from build123d import *

# Parameters (mm, degrees)
ESQUISSE1_W                  = 300
ESQUISSE1_H                  = 100
BOSS_EXTRU_1_DEPTH           = 1.5875
ESQUISSE2_W                  = 19.05
ESQUISSE2_H                  = 61.9
BOSS_EXTRU_2_DEPTH           = 1.5875
ESQUISSE3_W                  = 1.5875
ESQUISSE3_H                  = 61.9
BOSS_EXTRU_3_DEPTH           = 17.4625
ENL_V_MAT_EXTRU_1_REACH      = 5.175
ESQUISSE4_R                  = 1.5875
ENL_V_MAT_EXTRU_2_REACH      = 22.637
ESQUISSE5_R                  = 1.5875
ESQUISSE7_R                  = 1.5875
ENL_V_MAT_EXTRU_4_DEPTH      = 297.825
ENL_V_MAT_EXTRU_4_DEPTH_BACK = 4.175
ESQUISSE8_R                  = 1.5875
ENL_V_MAT_EXTRU_5_DEPTH      = 1.5875


with BuildPart() as part:
    # Esquisse1 → Boss.-Extru.1 (new body)
    with BuildSketch(Plane.XY):
        with Locations((29.89832913, 31.147540984)):
            Rectangle(ESQUISSE1_W, ESQUISSE1_H)
    extrude(amount=BOSS_EXTRU_1_DEPTH)

    # Esquisse2 → Boss.-Extru.2 (add)
    with BuildSketch(Plane(origin=(0, 0, 0), x_dir=(-1, 0, 0), z_dir=(0, 0, -1))):
        with Locations((108.98917087, 31.147540984)):
            Rectangle(ESQUISSE2_W, ESQUISSE2_H)
        with Locations((-168.78582913, 31.147540984)):
            Rectangle(ESQUISSE2_W, ESQUISSE2_H)
    extrude(amount=BOSS_EXTRU_2_DEPTH)

    # Esquisse3 → Boss.-Extru.3 (add)
    with BuildSketch(Plane(origin=(0, 0, -1.5875), x_dir=(-1, 0, 0), z_dir=(0, 0, -1))):
        with Locations((-177.51707913, 31.147540984)):
            Rectangle(ESQUISSE3_W, ESQUISSE3_H)
        with Locations((117.72042087, 31.147540984)):
            Rectangle(ESQUISSE3_W, ESQUISSE3_H)
    extrude(amount=BOSS_EXTRU_3_DEPTH)

    # Esquisse4 → Enlèv. mat.-Extru.1 (cut, up to next)
    with BuildSketch(Plane(origin=(0, 0, -1.5875), x_dir=(-1, 0, 0), z_dir=(0, 0, -1)), mode=Mode.PRIVATE) as enl_v_mat_extru_1_sk1:
        with Locations((-167.99207913, 52.572540984)):
            Circle(ESQUISSE4_R)
    enl_v_mat_extru_1_tool1 = extrude(enl_v_mat_extru_1_sk1.sketch, amount=-ENL_V_MAT_EXTRU_1_REACH, mode=Mode.PRIVATE) & part.part
    add(enl_v_mat_extru_1_tool1.solids().sort_by_distance((167.992079, 52.572541, -1.5875))[0], mode=Mode.SUBTRACT)
    # Esquisse4 → Enlèv. mat.-Extru.1 (cut, up to next)
    with BuildSketch(Plane(origin=(0, 0, -1.5875), x_dir=(-1, 0, 0), z_dir=(0, 0, -1)), mode=Mode.PRIVATE) as enl_v_mat_extru_1_sk2:
        with Locations((-167.99207913, 9.722540984)):
            Circle(ESQUISSE4_R)
    enl_v_mat_extru_1_tool2 = extrude(enl_v_mat_extru_1_sk2.sketch, amount=-ENL_V_MAT_EXTRU_1_REACH, mode=Mode.PRIVATE) & part.part
    add(enl_v_mat_extru_1_tool2.solids().sort_by_distance((167.992079, 9.722541, -1.5875))[0], mode=Mode.SUBTRACT)
    # Esquisse4 → Enlèv. mat.-Extru.1 (cut, up to next)
    with BuildSketch(Plane(origin=(0, 0, -1.5875), x_dir=(-1, 0, 0), z_dir=(0, 0, -1)), mode=Mode.PRIVATE) as enl_v_mat_extru_1_sk3:
        with Locations((108.19542087, 52.572540984)):
            Circle(ESQUISSE4_R)
    enl_v_mat_extru_1_tool3 = extrude(enl_v_mat_extru_1_sk3.sketch, amount=-ENL_V_MAT_EXTRU_1_REACH, mode=Mode.PRIVATE) & part.part
    add(enl_v_mat_extru_1_tool3.solids().sort_by_distance((-108.195421, 52.572541, -1.5875))[0], mode=Mode.SUBTRACT)
    # Esquisse4 → Enlèv. mat.-Extru.1 (cut, up to next)
    with BuildSketch(Plane(origin=(0, 0, -1.5875), x_dir=(-1, 0, 0), z_dir=(0, 0, -1)), mode=Mode.PRIVATE) as enl_v_mat_extru_1_sk4:
        with Locations((108.19542087, 9.722540984)):
            Circle(ESQUISSE4_R)
    enl_v_mat_extru_1_tool4 = extrude(enl_v_mat_extru_1_sk4.sketch, amount=-ENL_V_MAT_EXTRU_1_REACH, mode=Mode.PRIVATE) & part.part
    add(enl_v_mat_extru_1_tool4.solids().sort_by_distance((-108.195421, 9.722541, -1.5875))[0], mode=Mode.SUBTRACT)

    # Esquisse5 → Enlèv. mat.-Extru.2 (cut, up to next)
    with BuildSketch(Plane.XY.offset(1.5875), mode=Mode.PRIVATE) as enl_v_mat_extru_2_sk1:
        with Locations((-108.19542087, -8.533709016)):
            Circle(ESQUISSE5_R)
    enl_v_mat_extru_2_tool1 = extrude(enl_v_mat_extru_2_sk1.sketch, amount=-ENL_V_MAT_EXTRU_2_REACH, mode=Mode.PRIVATE) & part.part
    add(enl_v_mat_extru_2_tool1.solids().sort_by_distance((-108.195421, -8.533709, 1.5875))[0], mode=Mode.SUBTRACT)
    # Esquisse5 → Enlèv. mat.-Extru.2 (cut, up to next)
    with BuildSketch(Plane.XY.offset(1.5875), mode=Mode.PRIVATE) as enl_v_mat_extru_2_sk2:
        with Locations((-89.93917087, -8.533709016)):
            Circle(ESQUISSE5_R)
    enl_v_mat_extru_2_tool2 = extrude(enl_v_mat_extru_2_sk2.sketch, amount=-ENL_V_MAT_EXTRU_2_REACH, mode=Mode.PRIVATE) & part.part
    add(enl_v_mat_extru_2_tool2.solids().sort_by_distance((-89.939171, -8.533709, 1.5875))[0], mode=Mode.SUBTRACT)
    # Esquisse5 → Enlèv. mat.-Extru.2 (cut, up to next)
    with BuildSketch(Plane.XY.offset(1.5875), mode=Mode.PRIVATE) as enl_v_mat_extru_2_sk3:
        with Locations((-30.02042087, -8.533709016)):
            Circle(ESQUISSE5_R)
    enl_v_mat_extru_2_tool3 = extrude(enl_v_mat_extru_2_sk3.sketch, amount=-ENL_V_MAT_EXTRU_2_REACH, mode=Mode.PRIVATE) & part.part
    add(enl_v_mat_extru_2_tool3.solids().sort_by_distance((-30.020421, -8.533709, 1.5875))[0], mode=Mode.SUBTRACT)
    # Esquisse5 → Enlèv. mat.-Extru.2 (cut, up to next)
    with BuildSketch(Plane.XY.offset(1.5875), mode=Mode.PRIVATE) as enl_v_mat_extru_2_sk4:
        with Locations((29.89832913, -8.533709016)):
            Circle(ESQUISSE5_R)
    enl_v_mat_extru_2_tool4 = extrude(enl_v_mat_extru_2_sk4.sketch, amount=-ENL_V_MAT_EXTRU_2_REACH, mode=Mode.PRIVATE) & part.part
    add(enl_v_mat_extru_2_tool4.solids().sort_by_distance((29.898329, -8.533709, 1.5875))[0], mode=Mode.SUBTRACT)
    # Esquisse5 → Enlèv. mat.-Extru.2 (cut, up to next)
    with BuildSketch(Plane.XY.offset(1.5875), mode=Mode.PRIVATE) as enl_v_mat_extru_2_sk5:
        with Locations((89.81707913, -8.533709016)):
            Circle(ESQUISSE5_R)
    enl_v_mat_extru_2_tool5 = extrude(enl_v_mat_extru_2_sk5.sketch, amount=-ENL_V_MAT_EXTRU_2_REACH, mode=Mode.PRIVATE) & part.part
    add(enl_v_mat_extru_2_tool5.solids().sort_by_distance((89.817079, -8.533709, 1.5875))[0], mode=Mode.SUBTRACT)
    # Esquisse5 → Enlèv. mat.-Extru.2 (cut, up to next)
    with BuildSketch(Plane.XY.offset(1.5875), mode=Mode.PRIVATE) as enl_v_mat_extru_2_sk6:
        with Locations((149.73582913, -8.533709016)):
            Circle(ESQUISSE5_R)
    enl_v_mat_extru_2_tool6 = extrude(enl_v_mat_extru_2_sk6.sketch, amount=-ENL_V_MAT_EXTRU_2_REACH, mode=Mode.PRIVATE) & part.part
    add(enl_v_mat_extru_2_tool6.solids().sort_by_distance((149.735829, -8.533709, 1.5875))[0], mode=Mode.SUBTRACT)
    # Esquisse5 → Enlèv. mat.-Extru.2 (cut, up to next)
    with BuildSketch(Plane.XY.offset(1.5875), mode=Mode.PRIVATE) as enl_v_mat_extru_2_sk7:
        with Locations((167.99207913, -8.533709016)):
            Circle(ESQUISSE5_R)
    enl_v_mat_extru_2_tool7 = extrude(enl_v_mat_extru_2_sk7.sketch, amount=-ENL_V_MAT_EXTRU_2_REACH, mode=Mode.PRIVATE) & part.part
    add(enl_v_mat_extru_2_tool7.solids().sort_by_distance((167.992079, -8.533709, 1.5875))[0], mode=Mode.SUBTRACT)
    # Esquisse5 → Enlèv. mat.-Extru.2 (cut, up to next)
    with BuildSketch(Plane.XY.offset(1.5875), mode=Mode.PRIVATE) as enl_v_mat_extru_2_sk8:
        with Locations((167.99207913, 70.828790984)):
            Circle(ESQUISSE5_R)
    enl_v_mat_extru_2_tool8 = extrude(enl_v_mat_extru_2_sk8.sketch, amount=-ENL_V_MAT_EXTRU_2_REACH, mode=Mode.PRIVATE) & part.part
    add(enl_v_mat_extru_2_tool8.solids().sort_by_distance((167.992079, 70.828791, 1.5875))[0], mode=Mode.SUBTRACT)
    # Esquisse5 → Enlèv. mat.-Extru.2 (cut, up to next)
    with BuildSketch(Plane.XY.offset(1.5875), mode=Mode.PRIVATE) as enl_v_mat_extru_2_sk9:
        with Locations((149.73582913, 70.828790984)):
            Circle(ESQUISSE5_R)
    enl_v_mat_extru_2_tool9 = extrude(enl_v_mat_extru_2_sk9.sketch, amount=-ENL_V_MAT_EXTRU_2_REACH, mode=Mode.PRIVATE) & part.part
    add(enl_v_mat_extru_2_tool9.solids().sort_by_distance((149.735829, 70.828791, 1.5875))[0], mode=Mode.SUBTRACT)
    # Esquisse5 → Enlèv. mat.-Extru.2 (cut, up to next)
    with BuildSketch(Plane.XY.offset(1.5875), mode=Mode.PRIVATE) as enl_v_mat_extru_2_sk10:
        with Locations((89.81707913, 70.828790984)):
            Circle(ESQUISSE5_R)
    enl_v_mat_extru_2_tool10 = extrude(enl_v_mat_extru_2_sk10.sketch, amount=-ENL_V_MAT_EXTRU_2_REACH, mode=Mode.PRIVATE) & part.part
    add(enl_v_mat_extru_2_tool10.solids().sort_by_distance((89.817079, 70.828791, 1.5875))[0], mode=Mode.SUBTRACT)
    # Esquisse5 → Enlèv. mat.-Extru.2 (cut, up to next)
    with BuildSketch(Plane.XY.offset(1.5875), mode=Mode.PRIVATE) as enl_v_mat_extru_2_sk11:
        with Locations((29.89832913, 70.828790984)):
            Circle(ESQUISSE5_R)
    enl_v_mat_extru_2_tool11 = extrude(enl_v_mat_extru_2_sk11.sketch, amount=-ENL_V_MAT_EXTRU_2_REACH, mode=Mode.PRIVATE) & part.part
    add(enl_v_mat_extru_2_tool11.solids().sort_by_distance((29.898329, 70.828791, 1.5875))[0], mode=Mode.SUBTRACT)
    # Esquisse5 → Enlèv. mat.-Extru.2 (cut, up to next)
    with BuildSketch(Plane.XY.offset(1.5875), mode=Mode.PRIVATE) as enl_v_mat_extru_2_sk12:
        with Locations((-30.02042087, 70.828790984)):
            Circle(ESQUISSE5_R)
    enl_v_mat_extru_2_tool12 = extrude(enl_v_mat_extru_2_sk12.sketch, amount=-ENL_V_MAT_EXTRU_2_REACH, mode=Mode.PRIVATE) & part.part
    add(enl_v_mat_extru_2_tool12.solids().sort_by_distance((-30.020421, 70.828791, 1.5875))[0], mode=Mode.SUBTRACT)
    # Esquisse5 → Enlèv. mat.-Extru.2 (cut, up to next)
    with BuildSketch(Plane.XY.offset(1.5875), mode=Mode.PRIVATE) as enl_v_mat_extru_2_sk13:
        with Locations((-89.93917087, 70.828790984)):
            Circle(ESQUISSE5_R)
    enl_v_mat_extru_2_tool13 = extrude(enl_v_mat_extru_2_sk13.sketch, amount=-ENL_V_MAT_EXTRU_2_REACH, mode=Mode.PRIVATE) & part.part
    add(enl_v_mat_extru_2_tool13.solids().sort_by_distance((-89.939171, 70.828791, 1.5875))[0], mode=Mode.SUBTRACT)
    # Esquisse5 → Enlèv. mat.-Extru.2 (cut, up to next)
    with BuildSketch(Plane.XY.offset(1.5875), mode=Mode.PRIVATE) as enl_v_mat_extru_2_sk14:
        with Locations((-108.19542087, 70.828790984)):
            Circle(ESQUISSE5_R)
    enl_v_mat_extru_2_tool14 = extrude(enl_v_mat_extru_2_sk14.sketch, amount=-ENL_V_MAT_EXTRU_2_REACH, mode=Mode.PRIVATE) & part.part
    add(enl_v_mat_extru_2_tool14.solids().sort_by_distance((-108.195421, 70.828791, 1.5875))[0], mode=Mode.SUBTRACT)

    # Esquisse7 → Enlèv. mat.-Extru.4 (cut, two sides)
    with BuildSketch(Plane.ZY.offset(-176.72332913)) as enl_v_mat_extru_4_sk:
        with Locations((-10.31875, 52.572540984)):
            Circle(ESQUISSE7_R)
        with Locations((-10.31875, 9.722540984)):
            Circle(ESQUISSE7_R)
    extrude(amount=ENL_V_MAT_EXTRU_4_DEPTH, mode=Mode.SUBTRACT)
    extrude(enl_v_mat_extru_4_sk.sketch, amount=-ENL_V_MAT_EXTRU_4_DEPTH_BACK, mode=Mode.SUBTRACT)

    # Esquisse8 → Enlèv. mat.-Extru.5 (cut)
    with BuildSketch(Plane.XY.offset(1.5875)):
        with Locations((-20.06104587, 11.147540984)):
            Circle(ESQUISSE8_R)
        with Locations((-10.06104587, 11.147540984)):
            Circle(ESQUISSE8_R)
        with Locations((-0.06104587, 11.147540984)):
            Circle(ESQUISSE8_R)
        with Locations((9.93895413, 11.147540984)):
            Circle(ESQUISSE8_R)
        with Locations((19.93895413, 11.147540984)):
            Circle(ESQUISSE8_R)
        with Locations((-10.06104587, 21.147540984)):
            Circle(ESQUISSE8_R)
        with Locations((-0.06104587, 21.147540984)):
            Circle(ESQUISSE8_R)
        with Locations((9.93895413, 21.147540984)):
            Circle(ESQUISSE8_R)
        with Locations((19.93895413, 21.147540984)):
            Circle(ESQUISSE8_R)
        with Locations((-10.06104587, 31.147540984)):
            Circle(ESQUISSE8_R)
        with Locations((-0.06104587, 31.147540984)):
            Circle(ESQUISSE8_R)
        with Locations((9.93895413, 31.147540984)):
            Circle(ESQUISSE8_R)
        with Locations((19.93895413, 31.147540984)):
            Circle(ESQUISSE8_R)
        with Locations((-10.06104587, 41.147540984)):
            Circle(ESQUISSE8_R)
        with Locations((-0.06104587, 41.147540984)):
            Circle(ESQUISSE8_R)
        with Locations((9.93895413, 41.147540984)):
            Circle(ESQUISSE8_R)
        with Locations((19.93895413, 41.147540984)):
            Circle(ESQUISSE8_R)
        with Locations((-10.06104587, 51.147540984)):
            Circle(ESQUISSE8_R)
        with Locations((-0.06104587, 51.147540984)):
            Circle(ESQUISSE8_R)
        with Locations((9.93895413, 51.147540984)):
            Circle(ESQUISSE8_R)
        with Locations((19.93895413, 51.147540984)):
            Circle(ESQUISSE8_R)
        with Locations((-20.06104587, 21.147540984)):
            Circle(ESQUISSE8_R)
        with Locations((-20.06104587, 31.147540984)):
            Circle(ESQUISSE8_R)
        with Locations((-20.06104587, 41.147540984)):
            Circle(ESQUISSE8_R)
        with Locations((-20.06104587, 51.147540984)):
            Circle(ESQUISSE8_R)
    extrude(amount=-ENL_V_MAT_EXTRU_5_DEPTH, mode=Mode.SUBTRACT)


solid = part.part
Could you check a few things on this model? Use its own coordinates, in mm. A direction names the side the tool comes from. Give positions to 0.01 mm unless a question says otherwise; leave off trailing zeros. Order: outer loops, then holes, each group sorted by start corner. A loop starts at its lowest first (then second) coordinate and runs counter-clockwise, first axis right, second up. Notation, with made-up numbers: (-5, -5.5) - (32, -5.5) arc R18 cw to (32, 25.5) - close; hole circle Ø8 at (-18, 54.25). An arc over 180 degrees is marked (long way). Return JSON: item names as keys, results as strings. Group by question number.
Q1. Please list where these lines run through material, in increasing order: line 1 along X through (y, z) = (8, -0.25); line 2 along X through (y, z) = (6.5, -4); line 3 along Z through (x, y) = (-66.5, 15). Write a range as [from, to].
Q2. Will these pins go through, and if not, where does the flat tip stop? pin 1 Ø3 at (y, z) = (6.5, -10) entering from -X; pin 2 Ø12 at (x, z) = (97.5, -4) entering from -Y; pin 3 Ø0.5 at (y, z) = (35, -1) entering from +X; pin 4 Ø5 at (x, y) = (149.74, -8.53) entering from -Z.
Q3. Suppose I cut it at B-B, the plane y = 46. Please give me the cut outline in (x, z), and give its area (3 significant figures).
Q4. Suppose I cut it at A-A, the plane z = -16. Please give me the cut outline in (x, y).
Q5. Suppose I cut it at C-C, the plane x = -45.5. Please give me the cut outline in (y, z).
Q6. Which directions (+Z, -Z, +X, -X, +Y, -Y) give clear straight access to the entire face, cutting with the end or side of a thin tool? Please do faces 1 (the face through (-113, 0.198, -1)), 2 (the face through (168, 32, -1.588)), 3 (the face through (-113, 62.098, -1)).
Q7. Thinking about a two-plate mould opening in X: for faces 4 (the face through (177, 62.098, -5)), 5 (the face through (178.311, 31, -9)), 6 (the face through (176.723, 31, -10)), which applies, pulls with the +X half, pulls with the -X half, needs draft (parallel to the pull), parting line crosses it, or undercut?
Resolved:
{
 "1": {"line 1": "x = [-118.51, -99.46], [159.26, 178.31]", "line 2": "x = [-118.51, -116.93], [176.72, 178.31]", "line 3": "z = [0, 1.59]"},
 "2": {"pin 1": "stops at x = -118.51", "pin 2": "stops at y = -18.85", "pin 3": "stops at x = 178.31", "pin 4": "stops at z = 0"},
 "3": {"outline": "(-120.1, 0) - (-118.51, 0) - (-118.51, -19.05) - (-116.93, -19.05) - (-116.93, -1.59) - (-99.46, -1.59) - (-99.46, 0) - (159.26, 0) - (159.26, -1.59) - (176.72, -1.59) - (176.72, -19.05) - (178.31, -19.05) - (178.31, 0) - (179.9, 0) - (179.9, 1.59) - (-120.1, 1.59) - close", "area": "592 mm2"},
 "4": {"outline": "(-118.51, 0.2) - (-116.93, 0.2) - (-116.93, 62.1) - (-118.51, 62.1) - close; (176.72, 0.2) - (178.31, 0.2) - (178.31, 62.1) - (176.72, 62.1) - close"},
 "5": {"outline": "(-18.85, 0) - (81.15, 0) - (81.15, 1.59) - (-18.85, 1.59) - close"},
 "6": {"face 1": "-Z, +X, -X, -Y", "face 2": "-Z, +Y, -Y", "face 3": "-Z, +X, -X, +Y"},
 "7": {"face 4": "needs draft", "face 5": "pulls with the +X half", "face 6": "undercut"}
}
